Model file for the job. Use its own axes, mm. Coordinates: 2 decimals unless noted, no trailing zeros. Loops run counter-clockwise (first coordinate to the right, second up) from the corner with the lowest first, then second, coordinate; pieces in that order, holes last. Notation, with made-up numbers: (36, 85) -> (90, 85) arc R36 ccw to (90, 122) -> close; hole circle Ø4 at (44.25, -34.75). An arc over 180 degrees is marked (long way). Use one line per item in the form item = value.
```python
from build123d import *

# Parameters (mm, degrees)
BOSS_EXTRUDE1_DEPTH = 5
CUT_EXTRUDE1_DEPTH  = 64.006260456
FILLET2_R           = 2


# Read off the part's stored shape, not the designer's step: M4 Clearance Hole1
with BuildPart() as part:
    # Sketch1 → Boss-Extrude1 (new body)
    with BuildSketch(Plane(origin=(0, 0, 0), x_dir=(1, 0, 0), z_dir=(0, 1, 0))):
        with BuildLine():
            Line((-35, 0), (35, 0))
            ThreePointArc((35, 0), (41.5, 6.5), (35, 13))
            Line((35, 13), (2.949364905, 13))
            Line((2.949364905, 13), (2.949364905, 27.12))
            Line((2.949364905, 27.12), (-7.050635095, 27.12))
            Line((-7.050635095, 27.12), (-56.650635095, 20.149174599))
            Line((-56.650635095, 20.149174599), (-56.650635095, 12.5))
            Line((-56.650635095, 12.5), (-35, 0))
        make_face()
    extrude(amount=BOSS_EXTRUDE1_DEPTH)

    # M4 Clearance Hole1 outline → M4 Clearance Hole1 (revolve, cut)
    with BuildSketch(Plane(origin=(5, 0, -6.5), x_dir=(1, 0, 0), z_dir=(0, 0, 1))):
        Polygon((0, 0), (2.25, 0), (2.25, 4.979022509), (2.275, 5), (0, 5), align=None)
    revolve(axis=Axis((5, 0, -6.5), (0, 1, 0)), mode=Mode.SUBTRACT)

    # M4 Clearance Hole1 2 outline → M4 Clearance Hole1 2 (revolve, cut)
    with BuildSketch(Plane(origin=(35, 0, -6.5), x_dir=(1, 0, 0), z_dir=(0, 0, 1))):
        Polygon((0, 0), (2.25, 0), (2.25, 4.979022509), (2.275, 5), (0, 5), align=None)
    revolve(axis=Axis((35, 0, -6.5), (0, 1, 0)), mode=Mode.SUBTRACT)

    # Sketch4 → Cut-Extrude1 (cut, through all)
    with BuildSketch(Plane(origin=(0, 5, 0), x_dir=(1, 0, 0), z_dir=(0, 1, 0))):
        Polygon((-32.80827349, 23.5), (-7.050635095, 27.12), (-7.050635095, 15), (-32.80827349, 15), align=None)
    extrude(amount=-CUT_EXTRUDE1_DEPTH, mode=Mode.SUBTRACT)

    # Fillet2
    fillet2_edges = [part.edges().sort_by_distance(p)[0] for p in [
        (2.949364905, 2.5, -13),
        (-7.050635095, 2.5, -15),
        (-32.80827349, 2.5, -15),
    ]]
    fillet(fillet2_edges, radius=FILLET2_R)


solid = part.part
```
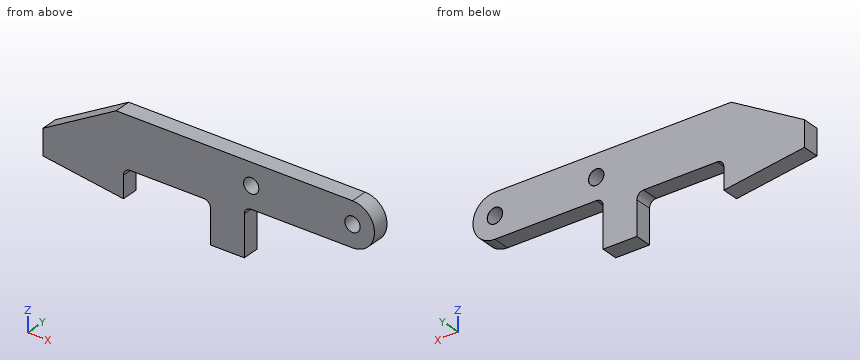
Q1. Band-saw the part on A-A, the plane y = 3.5. Write the cut outline in (x, z), and give its area (3 significant figures).
Result:
outline = (-56.65, -20.15) -> (-32.81, -23.5) -> (-32.81, -17) arc R2 cw to (-30.81, -15) -> (-9.05, -15) arc R2 cw to (-7.05, -17) -> (-7.05, -27.12) -> (2.95, -27.12) -> (2.95, -15) arc R2 cw to (4.95, -13) -> (35, -13) arc R6.5 ccw to (35, 0) -> (-35, 0) -> (-56.65, -12.5) -> close; hole circle Ø4.5 at (5, -6.5); hole circle Ø4.5 at (35, -6.5)
area = 1,500 mm2
Q2. Band-saw the part on D-D, the plane x = -40. Write the cut outline in (y, z), and give its area (3 significant figures).
Result:
outline = (0, -22.49) -> (5, -22.49) -> (5, -2.89) -> (0, -2.89) -> close
area = 98.0 mm2
Q3. Wall check: line 1 along Z through (x, y) = (35, 3.8); line 2 along X through (y, z) = (2.2, -6.5); line 3 along X through (y, z) = (2.5, -18.25). Give the ranges that are in metal, low to high.
Result:
line_1 = -13 to -8.75, -4.25 to 0
line_2 = -46.26 to 2.75, 7.25 to 32.75, 37.25 to 41.5
line_3 = -56.65 to -32.81, -7.05 to 2.95
Q4. Band-saw the part on C-C, the plane x = -16. Write the cut outline in (y, z), and give its area (3 significant figures).
Result:
outline = (0, -15) -> (5, -15) -> (5, 0) -> (0, 0) -> close
area = 75.0 mm2
Q5. Band-saw the part on B-B, the plane z = -6.5. Write the cut outline in (x, y) (3 decimals).
Result:
outline = (-46.258, 0) -> (2.75, 0) -> (2.75, 4.979) -> (2.725, 5) -> (-46.258, 5) -> close; (7.25, 0) -> (32.75, 0) -> (32.75, 4.979) -> (32.725, 5) -> (7.275, 5) -> (7.25, 4.979) -> close; (37.25, 0) -> (41.5, 0) -> (41.5, 5) -> (37.275, 5) -> (37.25, 4.979) -> close
Q6. Pin check, flat tips, straight feed: pin 1 Ø3 at (y, z) = (4, -12) entering from -X; pin 2 Ø1.5 at (x, y) = (12, 1.5) entering from -Z; pin 3 Ø2.5 at (x, y) = (-23.5, 3) entering from -Z. Stop position of each tip, or through.
Result:
pin_1 = -56.65
pin_2 = -13
pin_3 = -15
